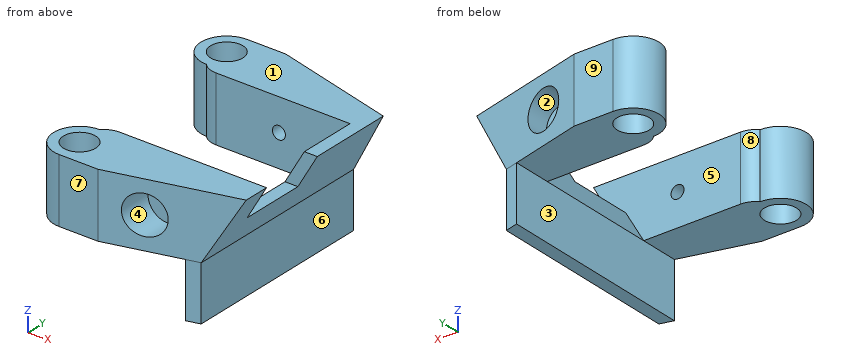
```python
from build123d import *

# Parameters (mm, degrees)
CROQUIS1_R              = 2.5
SALIENTE_EXTRUIR1_DEPTH = 10
CROQUIS2_R              = 1
CORTAR_EXTRUIR1_DEPTH   = 4
SALIENTE_EXTRUIR2_DEPTH = 13.5
CROQUIS4_R              = 3
CORTAR_EXTRUIR2_DEPTH   = 1
SALIENTE_EXTRUIR3_START = 5
CROQUIS6_R              = 3
SALIENTE_EXTRUIR3_DEPTH = 5
CORTAR_EXTRUIR3_DEPTH   = 10
SALIENTE_EXTRUIR4_DEPTH = 8.5
CROQUIS5_W              = 2
CROQUIS5_H              = 10
CORTAR_EXTRUIR4_DEPTH   = 6
REDONDEO1_R             = 3


with BuildPart() as part:
    # Croquis1 → Saliente-Extruir1 (new body)
    with BuildSketch(Plane.XY):
        with BuildLine():
            Line((-106.231635218, 22.700651543), (-131.231635218, 22.700651543))
            Line((-131.231635218, 22.700651543), (-131.231635218, 21.700651543))
            ThreePointArc((-131.231635218, 21.700651543), (-135.231635218, 17.700651543), (-131.231635218, 13.700651543))
            Line((-131.231635218, 13.700651543), (-125.231635218, 13.700651543))
            Line((-125.231635218, 13.700651543), (-125.231635218, 18.700651543))
            Line((-125.231635218, 18.700651543), (-106.231635218, 18.700651543))
            Line((-106.231635218, 18.700651543), (-106.231635218, 22.700651543))
        make_face()
        with Locations((-131.231635218, 17.700651543)):
            Circle(CROQUIS1_R, mode=Mode.SUBTRACT)
    extrude(amount=SALIENTE_EXTRUIR1_DEPTH)

    # Croquis2 → Cortar-Extruir1 (cut)
    with BuildSketch(Plane.XZ.offset(-18.700651543)):
        with Locations(Location((-119.231635218, 5, 0), (0, 0, 270))):
            Circle(CROQUIS2_R)
        Polygon((-106.231635218, 0), (-106.231635218, 10), (-112.00513791, 0), align=None)
    extrude(amount=-CORTAR_EXTRUIR1_DEPTH, mode=Mode.SUBTRACT)

    # Croquis3 → Saliente-Extruir2 (add)
    with BuildSketch(Plane.XZ.offset(-18.700651543)):
        Polygon((-106.231635218, 10), (-108.231635218, 10), (-114.00513791, 0), (-112.00513791, 0), align=None)
    extrude(amount=-SALIENTE_EXTRUIR2_DEPTH)

    # Croquis4 → Cortar-Extruir2 (cut)
    with BuildSketch(Plane.XZ.offset(-18.700651543)):
        with Locations(Location((-119.231635218, 5, 0), (0, 0, 270))):
            Circle(CROQUIS4_R)
    extrude(amount=-CORTAR_EXTRUIR2_DEPTH, mode=Mode.SUBTRACT)

    # Croquis6 → Saliente-Extruir3 (add)
    with BuildSketch(Plane.XZ.offset(-18.700651543).offset(SALIENTE_EXTRUIR3_START)):
        Polygon((-106.231635218, 10), (-125.231635218, 10), (-125.231635218, 0), (-112.00513791, 0), align=None)
        with Locations(Location((-119.231635218, 5, 0), (0, 0, 270))):
            Circle(CROQUIS6_R, mode=Mode.SUBTRACT)
    extrude(amount=-SALIENTE_EXTRUIR3_DEPTH)

    # Croquis7 → Cortar-Extruir3 (cut)
    with BuildSketch(Plane.XY.offset(10)):
        Polygon((-106.231635218, 18.700651543), (-106.231635218, 13.700651543), (-125.231635218, 13.700651543), align=None)
    extrude(amount=-CORTAR_EXTRUIR3_DEPTH, mode=Mode.SUBTRACT)

    # Croquis8 → Saliente-Extruir4 (add)
    with BuildSketch(Plane(origin=(0, 0, 0), x_dir=(-1, 0, 0), z_dir=(0, 0, -1))):
        Polygon((112.00513791, 17.181308729), (112.00513791, 32.200651543), (114.00513791, 32.200651543), (114.00513791, 16.65499294), align=None)
    extrude(amount=SALIENTE_EXTRUIR4_DEPTH)

    # Simetría1: part across plane


with BuildPart() as part_1:
    add(part.part)
    add(part.part.mirror(Plane(origin=(0, 32.200651543, 0), x_dir=(0, 0, 1), z_dir=(0, -1, 0))))

    # Croquis5 → Cortar-Extruir4 (cut, along a direction that is not the sketch's normal)
    with BuildSketch(Plane.XY.offset(10)):
        with Locations((-107.231635218, 27.700651543)):
            Rectangle(CROQUIS5_W, CROQUIS5_H)
    extrude(amount=-CORTAR_EXTRUIR4_DEPTH, dir=(0.49999999999999506, 0, 0.8660254037844416), mode=Mode.SUBTRACT)

    # Redondeo1
    # the kernel refuses this fillet: 3 mm, written as the material it takes off along each edge
    with BuildSketch(Plane(origin=(-131.231635218, 41.700651543, -5.590169944), x_dir=(1, 0, 0), z_dir=(0, 0, 1))) as redondeo1_piece_1:
        with BuildLine():
            CenterArc((2.236067977, 3), REDONDEO1_R, 221.810314896, 48.189685104)
            Line((0, 1), (-0.04472136, 0.96))
            ThreePointArc((-0.04472136, 0.96), (-0.06, 0.5), (-0.06, 0))
            Line((-0.06, 0), (0, -0.06))
            Line((0, -0.06), (2.236067977, -0.06))
            Line((2.236067977, -0.06), (2.236067977, 0))
        make_face()
    extrude(amount=21.180339887, mode=Mode.SUBTRACT)
    with BuildSketch(Plane(origin=(-131.231635218, 22.700651543, -5.590169944), x_dir=(0, -1, 0), z_dir=(0, 0, 1))) as redondeo1_piece_2:
        with BuildLine():
            CenterArc((3, 2.236067977), REDONDEO1_R, 180, 48.189685104)
            Line((0, 2.236067977), (-0.06, 2.236067977))
            Line((-0.06, 2.236067977), (-0.06, 0))
            Line((-0.06, 0), (0, -0.06))
            ThreePointArc((0, -0.06), (0.5, -0.06), (0.96, -0.04472136))
            Line((0.96, -0.04472136), (1, 0))
        make_face()
    extrude(amount=21.180339887, mode=Mode.SUBTRACT)


solid = part_1.part
```
Verification items for the finished model (mm, model axes). Face numbers are marked on the shaded views. A direction names the side the tool comes from. Coordinates: 2 decimals unless noted, no trailing zeros. Loops run counter-clockwise (first coordinate to the right, second up) from the corner with the lowest first, then second, coordinate; pieces in that order, holes last. Notation, with made-up numbers: (39.5, 27.5) -> (64.5, 27.5) arc R24 ccw to (64.5, 54.5) -> close; hole circle Ø11 at (3, 78). An arc over 180 degrees is marked (long way). Answer in a Markdown table with one row per item. Add a question column.
1. Section check D-D, the plane y = 38.5. Enter the section's corners in (x, z), then the cut area to 3 significant figures.
2. Draft check along Y on the marked faces 6, 7, 8 and 9. Enter one of: +Y half, -Y half, draft (parallel to the pull), parting line (faces both ways), or undercut.
3. Section check A-A, the plane z = 5.5. Give the number of separate pieces and of enclosed holes in the cut face, then the cut area to 3 significant figures.
4. Section check B-B, the plane x = -117.5. Enter the section's corners in (y, z).
5. Depth check by flat-ended pin: P1, Ø2, axis at x = -109.5, y = 29, coming from the +Z side; P2, Ø4, axis at y = 32, z = -2, coming from the -X side; P3, Ø5, axis at x = -114, z = 3.5, coming from the -Y side. Enter the tip coordinate at first touch or a pass-through.
6. Access from +Z, -Z, +X, -X, +Y, -Y to the whole of each face (thin tool, end or side, straight path). Record for the marked faces 1, 2, 3, 4 and 5.
7. Section check C-C, the plane x = -129.5. Enter the section's corners in (y, z).
8. Material ranges on probe 1 along Y at (x, z) = (-125.25, 4); probe 2 along Y at (x, z) = (-120.5, 4.75); probe 3 along X at (y, z) = (33.5, -1), recorded low to high. Write a range as [from, to].
Derived:
| question | item | result |
|---|---|---|
| 1 | outline | (-114.01, -8.5) -> (-112.01, -8.5) -> (-112.01, 0) -> (-106.23, 10) -> (-108.23, 10) -> (-114.01, 0) -> close |
| 1 | area | 37.0 mm² |
| 2 | face 6 | draft |
| 2 | face 7 | -Y half |
| 2 | face 8 | undercut |
| 2 | face 9 | +Y half |
| 3 | separate pieces | 4 |
| 3 | enclosed holes | 2 |
| 3 | area | 297 mm² |
| 4 | outline | (15.74, 0) -> (22.7, 0) -> (22.7, 10) -> (15.74, 10) -> (15.74, 7.45) -> (19.7, 7.45) -> (19.7, 2.55) -> (15.74, 2.55) -> close; (41.7, 0) -> (48.67, 0) -> (48.67, 2.55) -> (44.7, 2.55) -> (44.7, 7.45) -> (48.67, 7.45) -> (48.67, 10) -> (41.7, 10) -> close |
| 5 | P1 | stops at z = 4.8 |
| 5 | P2 | stops at x = -114.01 |
| 5 | P3 | stops at y = 16 |
| 6 | face 1 | +Z, +X, -X, +Y, -Y |
| 6 | face 2 | +Y |
| 6 | face 3 | -Z, -X, +Y, -Y |
| 6 | face 4 | -Y |
| 6 | face 5 | +Z, -X |
| 7 | outline | (13.7, 0) -> (15.9, 0) -> (15.9, 10) -> (13.7, 10) -> close; (19.5, 0) -> (22.66, 0) -> (22.66, 10) -> (19.5, 10) -> close; (41.74, 0) -> (44.9, 0) -> (44.9, 10) -> (41.74, 10) -> close; (48.5, 0) -> (50.7, 0) -> (50.7, 10) -> (48.5, 10) -> close |
| 8 | probe 1 | y = [13.7, 22.7], [41.7, 50.7] |
| 8 | probe 2 | y = [19.7, 22.7], [41.7, 44.7] |
| 8 | probe 3 | x = [-114.01, -112.01] |
